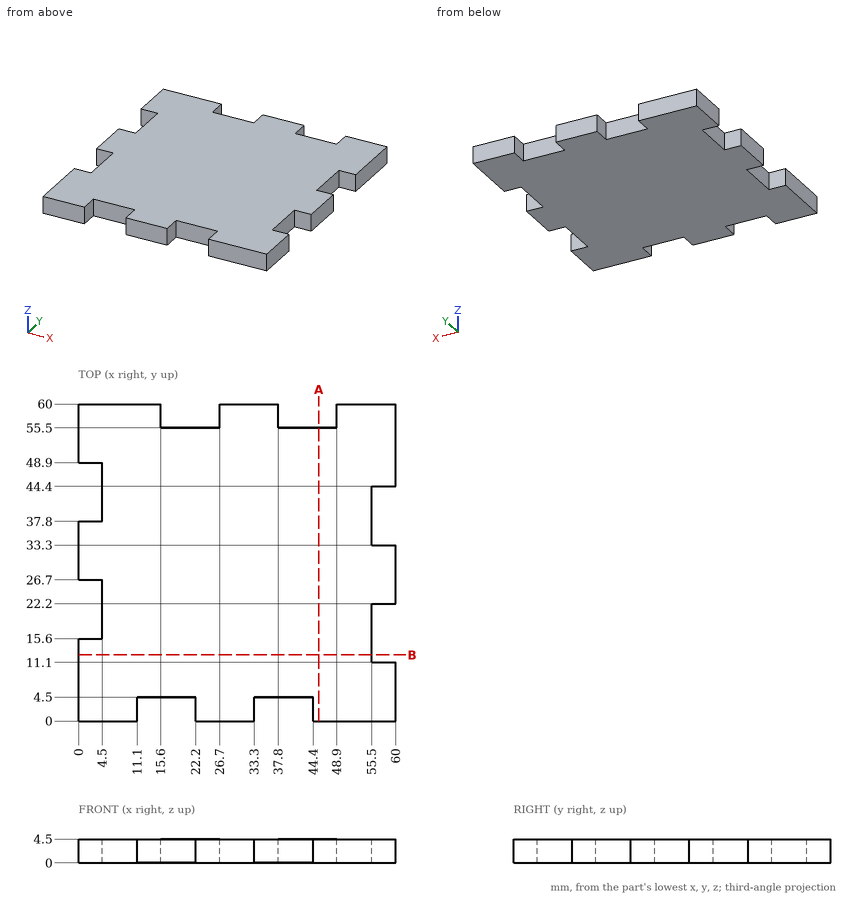
Input: dimensioned drawing with shaded views. Units: mm. Origin: part minimum x, y, z. Round coordinates to 2 decimals unless told otherwise and drop trailing zeros. Write each loop counter-clockwise with the first axis right and the second up, starting at its lowest first coordinate (ties: lowest second). Pieces come first, ordered by that corner, then holes. Notation, with made-up numbers: (26, -8) -> (67, -8) arc R25 cw to (67, 17) -> close; hole circle Ø8 at (3, -13). An arc over 180 degrees is marked (long way). Use CSV: the item, a comma, the result in double quotes. Start each with the question number.
Q1. Section A-A (x = 45.5). Return loops of the section in (y, z).
Q2. Line query: L1, parallel to Y at x = 4, z = 3.45; L2, parallel to Y at x = 57, z = 0.3; L3, parallel to X at y = 13, z = 0.65. Output: solid intervals per line, ascending.
Q3. First-contact query: pin 1 Ø2 at (y, z) = (35.5, 1) entering from +X; pin 2 Ø2 at (y, z) = (58.5, 1.5) entering from -X; pin 3 Ø1 at (y, z) = (18.5, 3) entering from -X; pin 4 Ø1.3 at (x, z) = (38.5, 2.5) entering from -Y. Flat tips, straight axial feed; report the tip coordinate or a pass-through.
Result sheet:
1,outline,"(0, 0) -> (55.5, 0) -> (55.5, 4.5) -> (0, 4.5) -> close"
2,L1,"0 to 15.6, 26.7 to 37.8, 48.9 to 60"
2,L2,"0 to 11.1, 22.2 to 33.3, 44.4 to 60"
2,L3,"0 to 55.5"
3,pin 1,"x = 55.5"
3,pin 2,"x = 0"
3,pin 3,"x = 4.5"
3,pin 4,"y = 4.5"
